Here's how the part is built. I have some questions about the finished solid (model axes, mm). A direction names the side the tool comes from. Coordinates: 2 decimals unless noted, no trailing zeros. Order: outer loops, then holes, each group sorted by start corner. A loop starts at its lowest first (then second) coordinate and runs counter-clockwise, first axis right, second up.
```python
from build123d import *

# Parameters (mm, degrees)
F0_W      = 29
F0_H      = 16.5
F1_DEPTH  = 38.5
F2_T      = -2
F3_DEPTH  = 2.25
F4_SIZE   = 2
F5_SIZE   = 2
F6_SIZE   = 1
F8_DEPTH  = 16.501
F10_DEPTH = 2
F11_R     = 2
F12_DEPTH = 2.001
F13_W     = 7.54
F13_H     = 7.25
F13_R     = 1.1
F14_DEPTH = 4.35
F15_W     = 5.538
F15_H     = 5.533
F17_W     = 5.538
F17_H     = 4.583


with BuildPart() as f1:
    # F0 (on Top) → F1 (new body)
    with BuildSketch(Plane.XY):
        with Locations((14.5, 8.25)):
            Rectangle(F0_W, F0_H)
    extrude(amount=F1_DEPTH)

    # F2
    f2_openings = [f1.faces().sort_by_distance(p)[0] for p in [
        (14.5, 8.25, 38.5),
    ]]
    offset(amount=F2_T, openings=f2_openings)

    # F3 (add): a face of the model
    f3_faces = [f1.faces().sort_by_distance(p)[0] for p in [
        (14.5, 8.25, 2),
    ]]
    extrude(f3_faces, amount=F3_DEPTH)

    # F4
    f4_edges = [f1.edges().sort_by_distance(p)[0] for p in [
        (29, 16.5, 19.25),
        (0, 16.5, 19.25),
        (0, 0, 19.25),
        (29, 0, 19.25),
    ]]
    chamfer(f4_edges, length=F4_SIZE)

    # F5 (call 1 of 4: OpenCascade refuses the feature's edges together)
    f5_edges = [f1.edges().sort_by_distance(p)[0] for p in [
        (0, 8.25, 0),
    ]]
    chamfer(f5_edges, length=F5_SIZE)

    # F5#2 (call 2 of 4)
    f5_2_edges = [f1.edges().sort_by_distance(p)[0] for p in [
        (14.5, 0, 0),
    ]]
    chamfer(f5_2_edges, length=F5_SIZE)

    # F5#3 (call 3 of 4)
    f5_3_edges = [f1.edges().sort_by_distance(p)[0] for p in [
        (29, 8.25, 0),
    ]]
    chamfer(f5_3_edges, length=F5_SIZE)

    # F5#4 (call 4 of 4)
    f5_4_edges = [f1.edges().sort_by_distance(p)[0] for p in [
        (14.5, 16.5, 0),
    ]]
    chamfer(f5_4_edges, length=F5_SIZE)

    # F6
    f6_edges = [f1.edges().sort_by_distance(p)[0] for p in [
        (14.5, 16.5, 38.5),
        (29, 8.25, 38.5),
        (14.5, 0, 38.5),
        (0, 8.25, 38.5),
        (1, 15.5, 38.5),
        (28, 15.5, 38.5),
        (28, 1, 38.5),
        (1, 1, 38.5),
    ]]
    chamfer(f6_edges, length=F6_SIZE)

    # F7 (on face) → F8 (cut, through all)
    with BuildSketch(Plane.XZ):
        Polygon((17.36, 12.834), (12.631, 12.834), (6.46, 8.664), (6.46, 4.94), (23.536, 4.94), (23.536, 8.664), align=None)
    extrude(amount=-F8_DEPTH, mode=Mode.SUBTRACT)

    # F9 (on face) → F10 (cut, through all)
    with BuildSketch(Plane.YZ.offset(29)):
        with BuildLine():
            ThreePointArc((5.0038961688, 23.1590909091), (8.1704306945, 19.7509741882), (11.5, 23))
            ThreePointArc((11.5, 23), (11.4990258118, 23.0795693055), (11.4961038312, 23.1590909091))
            ThreePointArc((11.4961038312, 23.1590909091), (8.25, 22.25), (5.0038961688, 23.1590909091))
        make_face()
        with BuildLine():
            ThreePointArc((5.0038961688, 23.1590909091), (8.25, 22.25), (11.4961038312, 23.1590909091))
            ThreePointArc((11.4961038312, 23.1590909091), (8.25, 26.25), (5.0038961688, 23.1590909091))
        make_face()
        with BuildLine():
            ThreePointArc((5.0038961688, 23.1590909091), (8.25, 26.25), (11.4961038312, 23.1590909091))
            ThreePointArc((11.4961038312, 23.1590909091), (13.6975062618, 25.4361502113), (14.5, 28.5))
            Line((14.5, 28.5), (2, 28.5))
            ThreePointArc((2, 28.5), (2.8024937382, 25.4361502113), (5.0038961688, 23.1590909091))
        make_face()
        with BuildLine():
            Line((2, 28.5), (14.5, 28.5))
            ThreePointArc((14.5, 28.5), (8.25, 34.75), (2, 28.5))
        make_face()
        with BuildLine():
            ThreePointArc((2, 28.5), (8.25, 34.75), (14.5, 28.5))
            Line((14.5, 28.5), (14.5, 38.5))
            Line((14.5, 38.5), (2, 38.5))
            Line((2, 38.5), (2, 28.5))
        make_face()
    extrude(amount=-F10_DEPTH, mode=Mode.SUBTRACT)

    # F11 (on face) → F12 (cut, through all)
    with BuildSketch(Plane.YZ.offset(2)):
        with Locations((8.25, 23)):
            Circle(F11_R)
    extrude(amount=-F12_DEPTH, mode=Mode.SUBTRACT)

    # F13 (on face) → F14 (join)
    with BuildSketch(Plane(origin=(27, 0, 0), x_dir=(0, -1, 0), z_dir=(-1, 0, 0))):
        with Locations((-8.25, 7.875)):
            Rectangle(F13_W, F13_H)
        with Locations((-8.25, 9)):
            Circle(F13_R, mode=Mode.SUBTRACT)
    extrude(amount=F14_DEPTH)

    # F15 (on face) → F18 section 0
    with BuildSketch(Plane.YZ.offset(29)):
        with Locations((8.25, 8.0385)):
            Rectangle(F15_W, F15_H)
    # F17 (on offset) → F18 section 1
    with BuildSketch(Plane.YZ.offset(24.55)):
        with Locations((8.25, 8.5135)):
            Rectangle(F17_W, F17_H)
    loft(mode=Mode.SUBTRACT)


solid = f1.part
```
Q1. If we section it at A-A on y = 8.25: Write out the boundary of the cut face in (x, z) (3 decimals), then the cut area to 3 significant figures.
Q2. If we section it at D-D on x = 21.5: Write out the boundary of the cut face in (y, z).
Q3. We'd pull the mould along Z, two halves only. Please class faces 1 (the flat face through (23.536, 15, 7)), 2 (the flat face through (27.512, 15.428, 37.896)), 3 (the flat face through (22.65, 8, 7)): pulls with the +Z half, pulls with the -Z half, needs draft (parallel to the pull), parting line crosses it, or undercut.
Q4. For faces 4 (the flat face through (9.59, 0.99, 10.78)), 5 (the cylindrical face through (23.613, 7.234, 8.579)), 6 (the flat face through (27, 8, 16)), 7 (the cylindrical face through (28.01, 2.78, 25.48)), which set-ups out of +Z, -Z, +X, -X, +Y, -Y let a thin tool reach every point of the face, with its end or its side?
Q5. If we section it at B-B on z = 14.5: Write out the boundary of the cut face in (x, y).
Q6. I need wall thicknesses on L1, parallel to Y at x = 24.15, z = 9; L2, parallel to Y at x = 24.75, z = 34.5; L3, parallel to X at y = 15.5, z = 5. Which ranges of each line are inside material? Lowest first, please.
Q7. If we section it at C-C on x = 5.5: Write out the boundary of the cut face in (y, z), then the cut area to 3 significant figures.
Q8. Will these pins go through, and if not, where does the flat tip stop? pin 1 (1 mm diameter, centred on y = 1, z = 6, fed in from +X); pin 2 (6 mm diameter, centred on x = 9.5, y = 6, fed in from +Z); pin 3 (1.4 mm diameter, centred on y = 7, z = 7.5, fed in from +X); pin 4 (6 mm diameter, centred on x = 8.5, y = 12.5, fed in from +Z).
Reply:
1. outline: (0, 2) - (2, 0) - (27, 0) - (29, 2) - (29, 5.272) - (24.55, 6.222) - (24.55, 7.9) - (22.65, 7.9) - (22.65, 4.25) - (2, 4.25) - (2, 21) - (0, 21) - close; (0, 25) - (2, 25) - (2, 38.5) - (1, 38.5) - (0, 37.5) - close; (22.65, 10.1) - (24.55, 10.1) - (24.55, 10.805) - (29, 10.805) - (29, 19.75) - (27, 19.75) - (27, 11.5) - (22.65, 11.5) - close
1. area: 215 mm2
2. outline: (0, 2) - (2, 0) - (14.5, 0) - (16.5, 2) - (16.5, 4.94) - (14.5, 4.94) - (14.5, 4.25) - (2, 4.25) - (2, 4.94) - (0, 4.94) - close; (0, 10.04) - (2, 10.04) - (2, 38.5) - (1, 38.5) - (0, 37.5) - close; (14.5, 10.04) - (16.5, 10.04) - (16.5, 37.5) - (15.5, 38.5) - (14.5, 38.5) - close
3. face 1: undercut
3. face 2: pulls with the +Z half
3. face 3: needs draft
4. face 4: +Y, -Y
4. face 5: +X
4. face 6: +Z
4. face 7: +Z, +X
5. outline: (0, 2) - (2, 0) - (27, 0) - (29, 2) - (29, 14.5) - (27, 16.5) - (2, 16.5) - (0, 14.5) - close; hole (2, 2) - (27, 2) - (27, 14.5) - (2, 14.5) - close
6. L1: y = 0 to 2, 4.48 to 7.15, 9.35 to 12.02, 14.5 to 16.5
6. L2: y = 0 to 2, 14.5 to 16.5
6. L3: x = 1 to 6.46, 23.54 to 28
7. outline: (0, 2) - (2, 0) - (14.5, 0) - (16.5, 2) - (16.5, 37.5) - (15.5, 38.5) - (14.5, 38.5) - (14.5, 4.25) - (2, 4.25) - (2, 38.5) - (1, 38.5) - (0, 37.5) - close
7. area: 202 mm2
8. pin 1: stops at x = 28.5
8. pin 2: stops at z = 4.25
8. pin 3: stops at x = 24.55
8. pin 4: stops at z = 38.5
